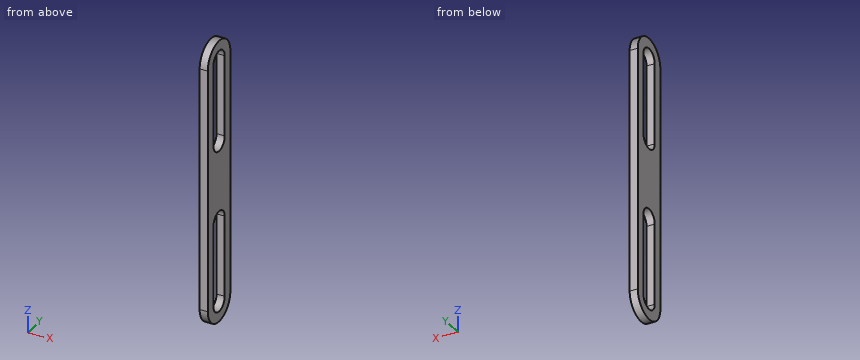
from build123d import *

# Parameters (mm, degrees)
BOSS_EXTRUDE1_DEPTH = 1.27
CUT_EXTRUDE1_DEPTH  = 3.54


with BuildPart() as part:
    # Sketch1 → Boss-Extrude1 (new body, symmetric)
    with BuildSketch(Plane(origin=(0, 0, 0), x_dir=(0, 0, -1), z_dir=(1, 0, 0))):
        with BuildLine():
            Line((-38.1, 6.35), (38.1, 6.35))
            ThreePointArc((38.1, 6.35), (44.45, 0), (38.1, -6.35))
            Line((38.1, -6.35), (-38.1, -6.35))
            ThreePointArc((-38.1, -6.35), (-44.45, 0), (-38.1, 6.35))
        make_face()
    extrude(amount=BOSS_EXTRUDE1_DEPTH, both=True)

    # Sketch2 → Cut-Extrude1 (cut, through all)
    with BuildSketch(Plane(origin=(1.27, 0, 0), x_dir=(0, 0, -1), z_dir=(1, 0, 0))):
        with BuildLine():
            Line((-38.1, 3.175), (-12.7, 3.175))
            ThreePointArc((-12.7, 3.175), (-9.525, 0), (-12.7, -3.175))
            Line((-12.7, -3.175), (-38.1, -3.175))
            ThreePointArc((-38.1, -3.175), (-41.275, 0), (-38.1, 3.175))
        make_face()
        with BuildLine():
            Line((38.1, 3.175), (12.7, 3.175))
            ThreePointArc((12.7, 3.175), (9.525, 0), (12.7, -3.175))
            Line((12.7, -3.175), (38.1, -3.175))
            ThreePointArc((38.1, -3.175), (41.275, 0), (38.1, 3.175))
        make_face()
    extrude(amount=-CUT_EXTRUDE1_DEPTH, mode=Mode.SUBTRACT)


solid = part.part
Could you check a few things on this model? Use its own coordinates, in mm. Round coordinates to 2 decimals unless told otherwise and drop trailing zeros. Write each loop counter-clockwise with the first axis right and the second up, starting at its lowest first coordinate (ties: lowest second). Pieces come first, ordered by that corner, then holes. Notation, with made-up numbers: (4.5, 63) -> (60.5, 63) arc R34 cw to (60.5, 95) -> close; hole circle Ø7 at (-39.5, 0). An arc over 180 degrees is marked (long way). Use a Markdown table: item, result.
1. If we section it at A-A (y = 0): List the corners of the cut face in (x, z) for me (3 decimals), then the cut area to 3 significant figures.
Answer key:
| item | result |
|---|---|
| outline | (-1.27, -44.45) -> (1.27, -44.45) -> (1.27, -41.275) -> (-1.27, -41.275) -> close; (-1.27, -9.525) -> (1.27, -9.525) -> (1.27, 9.525) -> (-1.27, 9.525) -> close; (-1.27, 41.275) -> (1.27, 41.275) -> (1.27, 44.45) -> (-1.27, 44.45) -> close |
| area | 64.5 mm^2 |
2. Please list where these lines run through material, in increasing order: probe 1 along Z at (x, y) = (0.2, 0) (3 decimals); probe 2 along Y at (x, z) = (-0.55, 33.5) (3 decimals); probe 3 along Z at (x, y) = (-1.15, 0.5).
Answer key:
| item | result |
|---|---|
| probe 1 | z = -44.45 to -41.275, -9.525 to 9.525, 41.275 to 44.45 |
| probe 2 | y = -6.35 to -3.175, 3.175 to 6.35 |
| probe 3 | z = -44.43 to -41.24, -9.56 to 9.56, 41.24 to 44.43 |
3. If we section it at B-B (x = 0.4): List the corners of the cut face in (y, z) for me (3 decimals).
Answer key:
| item | result |
|---|---|
| outline | (-6.35, -38.1) arc R6.35 ccw to (6.35, -38.1) -> (6.35, 38.1) arc R6.35 ccw to (-6.35, 38.1) -> close; hole (-3.175, -38.1) arc R3.175 ccw to (3.175, -38.1) -> (3.175, -12.7) arc R3.175 ccw to (-3.175, -12.7) -> close; hole (-3.175, 12.7) arc R3.175 ccw to (3.175, 12.7) -> (3.175, 38.1) arc R3.175 ccw to (-3.175, 38.1) -> close |
4. If we section it at C-C (z = -18.5): List the corners of the cut face in (x, y) for me (3 decimals).
Answer key:
| item | result |
|---|---|
| outline | (-1.27, -6.35) -> (1.27, -6.35) -> (1.27, -3.175) -> (-1.27, -3.175) -> close; (-1.27, 3.175) -> (1.27, 3.175) -> (1.27, 6.35) -> (-1.27, 6.35) -> close |
5. If we section it at D-D (z = 11): List the corners of the cut face in (x, y) for me, then the cut area to 3 significant figures.
Answer key:
| item | result |
|---|---|
| outline | (-1.27, -6.35) -> (1.27, -6.35) -> (1.27, -2.68) -> (-1.27, -2.68) -> close; (-1.27, 2.68) -> (1.27, 2.68) -> (1.27, 6.35) -> (-1.27, 6.35) -> close |
| area | 18.6 mm^2 |
